Check sheet for the modelled part. Datum: model origin and axes. Units: mm. A direction names the side the tool comes from. Round coordinates to 2 decimals unless told otherwise and drop trailing zeros. Order: outer loops, then holes, each group sorted by start corner. A loop starts at its lowest first (then second) coordinate and runs counter-clockwise, first axis right, second up. Notation, with made-up numbers: (7.25, 17) -> (25.25, 17) arc R17 ccw to (25.25, 24) -> close; hole circle Ø9 at (75, 29). An arc over 180 degrees is marked (long way). Use CSV: the item, a comma, the result in double quotes.
```python
from build123d import *

# Parameters (mm, degrees)
BOSS_EXTRU_1_DEPTH      = 6
ESQUISSE2_R             = 3
ESQUISSE2_R_2           = 1.5
ENL_V_MAT_EXTRU_1_DEPTH = 30
ENL_V_MAT_EXTRU_3_DEPTH = 10


with BuildPart() as part:
    # Esquisse1 → Boss.-Extru.1 (new body)
    with BuildSketch(Plane.XY):
        with BuildLine():
            Line((-14, 74), (-14, 80))
            Line((-14, 80), (-22, 80))
            Line((-22, 80), (-22, 0))
            Line((-22, 0), (-14, 0))
            Line((-14, 0), (-14, 6))
            Line((-14, 6), (-8, 6))
            Line((-8, 6), (-8, 0))
            Line((-8, 0), (0, 0))
            Line((0, 0), (0, 30))
            Line((0, 30), (20, 30))
            Line((20, 30), (20, 37))
            ThreePointArc((20, 37), (33, 50), (46, 37))
            Line((46, 37), (46, 30))
            Line((46, 30), (66, 30))
            Line((66, 30), (66, 0))
            Line((66, 0), (74, 0))
            Line((74, 0), (74, 6))
            Line((74, 6), (80, 6))
            Line((80, 6), (80, 0))
            Line((80, 0), (88, 0))
            Line((88, 0), (88, 80))
            Line((88, 80), (80, 80))
            Line((80, 80), (80, 74))
            Line((80, 74), (74, 74))
            Line((74, 74), (74, 80))
            Line((74, 80), (66, 80))
            Line((66, 80), (66, 60))
            Line((66, 60), (0, 60))
            Line((0, 60), (0, 80))
            Line((0, 80), (-8, 80))
            Line((-8, 80), (-8, 74))
            Line((-8, 74), (-14, 74))
        make_face()
    extrude(amount=BOSS_EXTRU_1_DEPTH)

    # Esquisse2 → Enlèv. mat.-Extru.1 (cut)
    with BuildSketch(Plane.XY.offset(6)):
        with Locations((-11, 31)):
            Circle(ESQUISSE2_R)
        with Locations((-11, 14)):
            Circle(ESQUISSE2_R_2)
    extrude(amount=-ENL_V_MAT_EXTRU_1_DEPTH, mode=Mode.SUBTRACT)

    # Esquisse5 → Enlèv. mat.-Extru.3 (cut)
    with BuildSketch(Plane.XY.offset(6)):
        Polygon((77, 74), (77, 6), (80, 6), (80, 0), (88, 0), (88, 80), (80, 80), (80, 74), align=None)
    extrude(amount=-ENL_V_MAT_EXTRU_3_DEPTH, mode=Mode.SUBTRACT)


solid = part.part
```
Q1. Sectioned sample at A-A, the plane x = -11. Enter the section's corners in (y, z), then the cut area to 3 significant figures.
Result sheet:
outline,"(6, 0) -> (12.5, 0) -> (12.5, 6) -> (6, 6) -> close; (15.5, 0) -> (28, 0) -> (28, 6) -> (15.5, 6) -> close; (34, 0) -> (74, 0) -> (74, 6) -> (34, 6) -> close"
area,"354 mm^2"
Q2. Scan lines: L1, parallel to Y at x = -11, z = 2.3; L2, parallel to X at y = 4.5, z = 5.3; L3, parallel to X at y = 62, z = 0.5. Record each from-to range of solid material in increasing order.
Result sheet:
L1,"y = 6 to 12.5, 15.5 to 28, 34 to 74"
L2,"x = -22 to -14, -8 to 0, 66 to 74"
L3,"x = -22 to 0, 66 to 77"
Q3. Sectioned sample at C-C, the plane z = 1.8. State how many separate pieces and enclosed holes the cut face has, then the cut area to 3 significant figures.
Result sheet:
separate pieces,"1"
enclosed holes,"2"
area,"4,030 mm^2"
Q4. Mould release check, pull along Y, two halves, no side actions. Record for faces 5 (the face through (-11, 6, 3)), 6 (the face through (-12.5, 14.07, 3.04)), 7 (the face through (70, 80, 3)), 8 (the face through (27, 49, 6)): pulls with the +Y half, pulls with the -Y half, needs draft (parallel to the pull), parting line crosses it, or undercut.
Result sheet:
face 5,"pulls with the -Y half"
face 6,"undercut"
face 7,"pulls with the +Y half"
face 8,"needs draft"
Q5. Sectioned sample at B-B, the plane y = 14. Enter the section's corners in (x, z), then the cut area to 3 significant figures.
Result sheet:
outline,"(-22, 0) -> (-12.5, 0) -> (-12.5, 6) -> (-22, 6) -> close; (-9.5, 0) -> (0, 0) -> (0, 6) -> (-9.5, 6) -> close; (66, 0) -> (77, 0) -> (77, 6) -> (66, 6) -> close"
area,"180 mm^2"
Q6. Access from +Z, -Z, +X, -X, +Y, -Y to the whole of each face (thin tool, end or side, straight path). Record for faces 1 (the face through (-8, 3, 3)), 2 (the face through (-13.21, 33.03, 3.04)), 3 (the face through (76, 74, 3)), 4 (the face through (-14, 77, 3)).
Result sheet:
face 1,"+Z, -Z, -Y"
face 2,"+Z, -Z"
face 3,"+Z, -Z, +X, +Y"
face 4,"+Z, -Z, +Y"
Q7. Go/stop test with flat-tipped pins: pin 1 (8 mm diameter, centred on x = -11, y = 31, fed in from +Z); pin 2 (2 mm diameter, centred on x = 32.5, z = 2.5, fed in from -Y); pin 3 (3 mm diameter, centred on y = 3, z = 2, fed in from +X); pin 4 (3 mm diameter, centred on x = 6, z = 3, fed in from -Y). Record where each tip stops, or that it passes through.
Result sheet:
pin 1,"stops at z = 6"
pin 2,"stops at y = 49.91"
pin 3,"stops at x = 74"
pin 4,"stops at y = 30"
Q8. Sectioned sample at D-D, the plane y = 24. Enter the section's corners in (x, z), then the cut area to 3 significant figures.
Result sheet:
outline,"(-22, 0) -> (0, 0) -> (0, 6) -> (-22, 6) -> close; (66, 0) -> (77, 0) -> (77, 6) -> (66, 6) -> close"
area,"198 mm^2"
